Could you check a few things on this model? Use its own coordinates, in mm. Face numbers are marked on the shaded views. A direction names the side the tool comes from. Give positions to 0.01 mm unless a question says otherwise; leave off trailing zeros. Loops run counter-clockwise (first coordinate to the right, second up) from the corner with the lowest first, then second, coordinate; pieces in that order, holes last. Notation, with made-up numbers: (-20, 43) - (-7, 43) arc R36 ccw to (-7, 81) - close; hole circle Ø7 at (37.25, 40.25). An arc over 180 degrees is marked (long way). One line per item, written item: value. Start each with the question number.
Q1. If we mould it in two halves opening along X, with no side actions, what happens to the marked faces 1, 2 and 3? For each: released by +X, released by -X, zero draft, split by the parting line, or undercut.
Q2. If I drill on line 1 (Z direction, x = -40, y = 17); line 2 (Z direction, x = 4, y = -21); line 3 (X direction, y = 25.5, z = 4.5), over which ranges is the centre line in solid material (lowest first)? Write a range as from..to.
Q3. I want a section at A-A (y = 0). Please give me the cut outline in (x, z), then the cut area to 3 significant figures.
Q4. I want a section at C-C (x = -38). Please give me the cut outline in (y, z).
Q5. I want a section at B-B (z = 14.5). Please give me the cut outline in (x, y).
Q6. I want a section at D-D (z = -3.5). Please give me the cut outline in (x, y), then the cut area to 3 significant figures.
Q7. For the marked faces 4, 5 and 6, which set-ups out of +Z, -Z, +X, -X, +Y, -Y let a thin tool reach every point of the face, with its end or its side?
Q8. I'm going to push flat-ended pins straight in: P1, Ø2, axis at x = 0.5, y = -26.5, coming from the -Z side; P2, Ø4, axis at x = 10, y = -37, coming from the +Z side; P3, Ø10, axis at y = 6.5, z = 9, coming from the +X side. Where does each tip first touch, or does it pass through?
```python
from build123d import *

# Parameters (mm, degrees)
CROQUIS2_R              = 47.5
CROQUIS2_R_2            = 5.5
SALIENTE_EXTRUIR1_DEPTH = 10
CROQUIS2_4_R            = 5.5
SALIENTE_EXTRUIR2_DEPTH = 20
CROQUIS6_R              = 5
SALIENTE_EXTRUIR3_DEPTH = 10


with BuildPart() as part:
    # Croquis2 → Saliente-Extruir1 (new body)
    with BuildSketch(Plane.XY):
        Circle(CROQUIS2_R)
        with Locations((-38, 0)):
            Circle(CROQUIS2_R_2, mode=Mode.SUBTRACT)
        with BuildLine():
            ThreePointArc((-19, -19.183326093), (27, 0), (-19, 19.183326093))
            ThreePointArc((-19, 19.183326093), (-11, 0), (-19, -19.183326093))
        make_face(mode=Mode.SUBTRACT)
    extrude(amount=SALIENTE_EXTRUIR1_DEPTH)

    # Croquis2_4 → Saliente-Extruir2 (add)
    with BuildSketch(Plane.XY):
        with Locations((-38, 0)):
            Circle(CROQUIS2_4_R)
        with BuildLine():
            ThreePointArc((-19, -19.183326093), (-11, 0), (-19, 19.183326093))
            ThreePointArc((-19, 19.183326093), (27, 0), (-19, -19.183326093))
        make_face()
    extrude(amount=SALIENTE_EXTRUIR2_DEPTH)

    # Croquis6 → Saliente-Extruir3 (add)
    with BuildSketch(Plane(origin=(0, 0, 0), x_dir=(-1, 0, 0), z_dir=(0, 0, -1))):
        with Locations(Location((0, 0, 0), (0, 0, 180))):
            Circle(CROQUIS6_R)
    extrude(amount=SALIENTE_EXTRUIR3_DEPTH)


solid = part.part
```
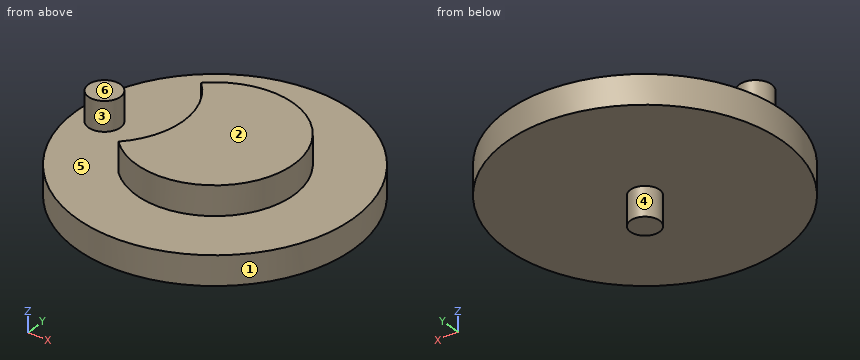
Worked answers:
1. face 1: split by the parting line
1. face 2: zero draft
1. face 3: undercut
2. line 1: z = 0..10
2. line 2: z = 0..20
2. line 3: x = -40.07..40.07
3. outline: (-47.5, 0) - (-5, 0) - (-5, -10) - (5, -10) - (5, 0) - (47.5, 0) - (47.5, 10) - (27, 10) - (27, 20) - (-11, 20) - (-11, 10) - (-32.5, 10) - (-32.5, 20) - (-43.5, 20) - (-43.5, 10) - (-47.5, 10) - close
3. area: 1,540 mm²
4. outline: (-28.5, 0) - (28.5, 0) - (28.5, 10) - (5.5, 10) - (5.5, 20) - (-5.5, 20) - (-5.5, 10) - (-28.5, 10) - close
5. outline: circle Ø11 at (-38, 0); (-19, -19.18) arc R27 ccw (long way) to (-19, 19.18) arc R27 cw to start
6. outline: circle Ø10 at (0, 0)
6. area: 78.5 mm²
7. face 4: -Z
7. face 5: +Z
7. face 6: +Z, +X, -X, +Y, -Y
8. P1: stops at z = 0
8. P2: stops at z = 10
8. P3: stops at x = 47.48
